Here's how the part is built. I have some questions about the finished solid (model axes, mm). Face numbers are marked on the shaded views. A direction names the side the tool comes from. Round coordinates to 2 decimals unless told otherwise and drop trailing zeros. Write each loop counter-clockwise with the first axis right and the second up, starting at its lowest first coordinate (ties: lowest second). Pieces come first, ordered by that corner, then holes. Notation, with made-up numbers: (-19, 8) -> (-4, 8) arc R8 cw to (-4, 18) -> close; hole circle Ø9 at (80.5, -34.75). An arc over 180 degrees is marked (long way). Put each result on its own line as item: value. Start each with the question number.
1) We'd pull the mould along X, two halves only. Please class the marked faces 1, 2 and 3: released by +X, released by -X, zero draft, split by the parting line, or undercut.
2) I want a section at A-A, the plane x = 0. List the corners of the cut face in (y, z) for me.
3) If I drill on line 1 along X through (y, z) = (3.25, 0); line 2 along Y through (x, z) = (25.5, -4); line 3 along X through (y, z) = (5.55, -7.5), over which ranges is the centre line in solid material (lowest first)? Write a range as [from, to].
4) I want a section at B-B, the plane z = 0. List the corners of the cut face in (x, y) for me.
5) Which directions (+Z, -Z, +X, -X, +Y, -Y) give clear straight access to the entire face, cutting with the end or side of a thin tool? Please do the marked faces 4 and 5.
6) I want a section at D-D, the plane z = -7.5. List the corners of the cut face in (x, y) for me.
7) I want a section at C-C, the plane z = 15. List the corners of the cut face in (x, y) for me, then the cut area to 3 significant figures.
8) Will these pins go through, and if not, where does the flat tip stop? P1, Ø1.5, axis at y = 4, z = -13.5, coming from the +X side; P2, Ø5, axis at x = -12.99, z = -7.5, coming from the -Y side; P3, Ø1.5, axis at y = 4, z = 6.5, coming from the -X side; P4, Ø6.5, axis at x = 12.99, z = -7.5, coming from the +Y side.
from build123d import *

# Parameters (mm, degrees)
SKETCH1_R           = 24.8
BOSS_EXTRUDE1_DEPTH = 3.1
SKETCH2_R           = 35
BOSS_EXTRUDE2_DEPTH = 2.6
SKETCH3_R           = 20.05
CUT_EXTRUDE1_DEPTH  = 5
CUT_EXTRUDE2_REACH  = 51.749
SKETCH4_R           = 2.1


with BuildPart() as part:
    # Sketch1 → Boss-Extrude1 (new body)
    with BuildSketch(Plane(origin=(0, 0, 0), x_dir=(1, 0, 0), z_dir=(0, 1, 0))):
        with Locations(Location((0, 0, 0), (0, 0, 90))):
            Circle(SKETCH1_R)
    extrude(amount=BOSS_EXTRUDE1_DEPTH)

    # Sketch2 → Boss-Extrude2 (add)
    with BuildSketch(Plane(origin=(0, 3.1, 0), x_dir=(1, 0, 0), z_dir=(0, 1, 0))):
        with Locations(Location((0, 0, 0), (0, 0, 270))):
            Circle(SKETCH2_R)
    extrude(amount=BOSS_EXTRUDE2_DEPTH)

    # Sketch3 → Cut-Extrude1 (cut)
    with BuildSketch(Plane.XZ):
        with Locations(Location((0, 0, 0), (0, 0, 270))):
            Circle(SKETCH3_R)
    extrude(amount=-CUT_EXTRUDE1_DEPTH, mode=Mode.SUBTRACT)

    # Sketch4 → Cut-Extrude2 (cut, up to next)
    with BuildSketch(Plane.XZ.offset(-5), mode=Mode.PRIVATE) as cut_extrude2_sk1:
        with Locations(Location((0, 15, 0), (0, 0, 270))):
            Circle(SKETCH4_R)
    cut_extrude2_tool1 = extrude(cut_extrude2_sk1.sketch, amount=-CUT_EXTRUDE2_REACH, mode=Mode.PRIVATE) & part.part
    # Sketch4 → Cut-Extrude2 (cut, up to next)
    with BuildSketch(Plane.XZ.offset(-5), mode=Mode.PRIVATE) as cut_extrude2_sk2:
        with Locations(Location((-12.990381057, -7.5, 0), (0, 0, 270))):
            Circle(SKETCH4_R)
    cut_extrude2_tool2 = extrude(cut_extrude2_sk2.sketch, amount=-CUT_EXTRUDE2_REACH, mode=Mode.PRIVATE) & part.part
    # Sketch4 → Cut-Extrude2 (cut, up to next)
    with BuildSketch(Plane.XZ.offset(-5), mode=Mode.PRIVATE) as cut_extrude2_sk3:
        with Locations(Location((12.990381057, -7.5, 0), (0, 0, 270))):
            Circle(SKETCH4_R)
    cut_extrude2_tool3 = extrude(cut_extrude2_sk3.sketch, amount=-CUT_EXTRUDE2_REACH, mode=Mode.PRIVATE) & part.part
    add(cut_extrude2_tool1.solids().sort_by_distance((0, 5, 15))[0], mode=Mode.SUBTRACT)
    add(cut_extrude2_tool2.solids().sort_by_distance((-12.990381, 5, -7.5))[0], mode=Mode.SUBTRACT)
    add(cut_extrude2_tool3.solids().sort_by_distance((12.990381, 5, -7.5))[0], mode=Mode.SUBTRACT)


solid = part.part
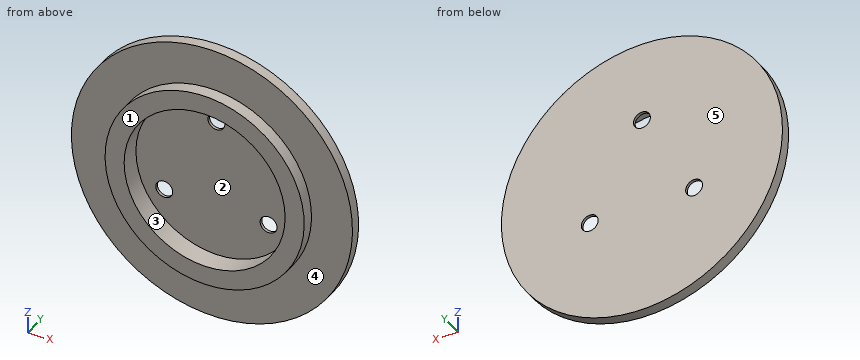
Findings:
1. face 1: zero draft
1. face 2: undercut
1. face 3: undercut
2. outline: (0, -24.8) -> (3.1, -24.8) -> (3.1, -35) -> (5.7, -35) -> (5.7, 12.9) -> (5, 12.9) -> (5, -20.05) -> (0, -20.05) -> close; (0, 20.05) -> (5, 20.05) -> (5, 17.1) -> (5.7, 17.1) -> (5.7, 35) -> (3.1, 35) -> (3.1, 24.8) -> (0, 24.8) -> close
3. line 1: x = [-35, -20.05], [20.05, 35]
3. line 2: y = [3.1, 5.7]
3. line 3: x = [-34.19, -15.09], [-10.89, 10.89], [15.09, 34.19]
4. outline: (-35, 3.1) -> (-24.8, 3.1) -> (-24.8, 0) -> (-20.05, 0) -> (-20.05, 5) -> (20.05, 5) -> (20.05, 0) -> (24.8, 0) -> (24.8, 3.1) -> (35, 3.1) -> (35, 5.7) -> (-35, 5.7) -> close
5. face 4: -Y
5. face 5: +Z, -Z, +X, -X, +Y
6. outline: (-34.19, 3.1) -> (-23.64, 3.1) -> (-23.64, 0) -> (-18.59, 0) -> (-18.59, 5) -> (-15.09, 5) -> (-15.09, 5.7) -> (-34.19, 5.7) -> close; (-10.89, 5) -> (10.89, 5) -> (10.89, 5.7) -> (-10.89, 5.7) -> close; (15.09, 5) -> (18.59, 5) -> (18.59, 0) -> (23.64, 0) -> (23.64, 3.1) -> (34.19, 3.1) -> (34.19, 5.7) -> (15.09, 5.7) -> close
7. outline: (-31.62, 3.1) -> (-19.75, 3.1) -> (-19.75, 0) -> (-13.3, 0) -> (-13.3, 5) -> (-2.1, 5) -> (-2.1, 5.7) -> (-31.62, 5.7) -> close; (2.1, 5) -> (13.3, 5) -> (13.3, 0) -> (19.75, 0) -> (19.75, 3.1) -> (31.62, 3.1) -> (31.62, 5.7) -> (2.1, 5.7) -> close
7. area: 151 mm2
8. P1: stops at x = 32.6
8. P2: stops at y = 5
8. P3: stops at x = -34.52
8. P4: stops at y = 5.7
